Geometry: final body of the model. Coordinates: model frame, mm. Face numbers are marked on the shaded views. A direction names the side the tool comes from. Coordinates: 2 decimals unless noted, no trailing zeros. Order: outer loops, then holes, each group sorted by start corner. A loop starts at its lowest first (then second) coordinate and runs counter-clockwise, first axis right, second up. Notation, with made-up numbers: M 17.25,-25.5 L 27.25,-25.5 A26 ccw 27.25,-3.5 Z; hole C 48,40.5 d7. An arc over 180 degrees is marked long. Write item = value, one per line.
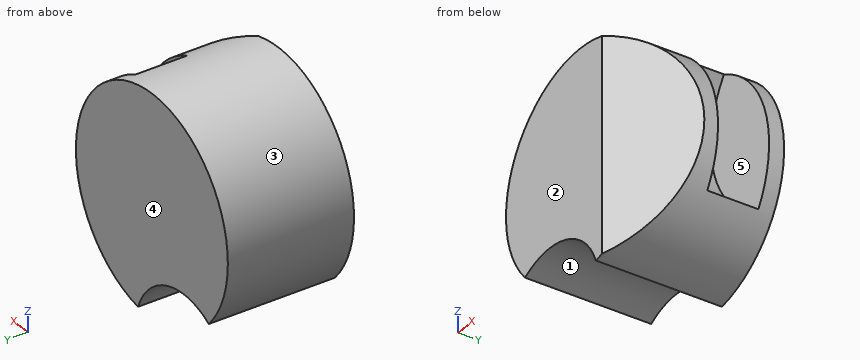
from build123d import *

# Parameters (mm, degrees)
BOSS_EXTRUDE1_DEPTH = 84
CUT_EXTRUDE2_DEPTH  = 34
CUT_EXTRUDE3_DEPTH  = 144.7823905
CUT_EXTRUDE4_DEPTH  = 43


with BuildPart() as part:
    # Sketch1 → Boss-Extrude1 (new body)
    with BuildSketch(Plane(origin=(0, 0, 0), x_dir=(1, 0, 0), z_dir=(0, 1, 0))):
        with BuildLine():
            ThreePointArc((-54.355236912, 47.976642444), (23.634324541, -68.539541168), (13.231432449, 71.2823905))
            ThreePointArc((13.231432449, 71.2823905), (-15.004428567, 43.512842845), (-54.355236912, 47.976642444))
        make_face()
    extrude(amount=BOSS_EXTRUDE1_DEPTH)

    # Sketch3 → Cut-Extrude2 (cut)
    with BuildSketch(Plane(origin=(0, 74, 0), x_dir=(1, 0, 0), z_dir=(0, 1, 0))):
        with BuildLine():
            ThreePointArc((62.290772837, 37.095951523), (20.191041077, -6.413624813), (29.465733324, -66.242135833))
            ThreePointArc((29.465733324, -66.242135833), (69.097787087, -21.948708839), (62.290772837, 37.095951523))
        make_face()
    extrude(amount=-CUT_EXTRUDE2_DEPTH, mode=Mode.SUBTRACT)

    # Sketch9 → Cut-Extrude3 (cut, through all)
    with BuildSketch(Plane.XY.offset(72.5)):
        Polygon((72.5, 30.908380348), (18.965114857, 0), (72.5, 0), align=None)
    extrude(amount=-CUT_EXTRUDE3_DEPTH, mode=Mode.SUBTRACT)

    # Sketch10 → Cut-Extrude4 (cut)
    with BuildSketch(Plane(origin=(0, 63, 0), x_dir=(1, 0, 0), z_dir=(0, 1, 0))):
        Polygon((-3.366442431, -32.270509831), (7.531695489, 1.270509831), (-21, 22), (-49.531695489, 1.270509831), (-38.633557569, -32.270509831), align=None)
    extrude(amount=-CUT_EXTRUDE4_DEPTH, mode=Mode.SUBTRACT)


solid = part.part
1) Mould query, pull axis X, two halves, no side actions, for the marked faces 1, 2 and 3. Classes: pulls with the +X half, pulls with the -X half, needs draft (parallel to the pull), parting line crosses it, or undercut.
Numbers:
face_1 = undercut
face_2 = needs draft
face_3 = parting line crosses it
2) Pin query (flat end, axial travel): pin 1 (2 mm diameter, centred on y = 66.5, z = -50, fed in from -X); pin 2 (17.5 mm diameter, centred on x = -23.5, y = 42, fed in from -Z); pin 3 (3 mm diameter, centred on x = 43.5, y = 47.5, fed in from -Z). Return the tip coordinate at first contact, or that it passes through.
Numbers:
pin_1 = -4.08
pin_2 = -43.6
pin_3 = -59.1
3) Section D-D, the plane x = 51. Return loops of the section in (y, z).
Numbers:
outline = M 18.5,-51.53 L 84,-51.53 L 84,51.53 L 74,51.53 L 74,-31.89 L 40,-31.89 L 40,51.53 L 18.5,51.53 Z
4) Set-up query: the marked faces 4 and 5. Return all of +Z, -Z, +X, -X, +Y, -Y with unobstructed straight access to the full face (end or side cutting, diameter ignored); none if empty.
Numbers:
face_4 = +Z, -Z, +X, -X, +Y
face_5 = +X
5) Section A-A, the plane x = 0. Return loops of the section in (y, z), and give its area (3 significant figures).
Numbers:
outline = M 0,-52.13 L 84,-52.13 L 84,72.5 L 0,72.5 Z; hole M 20,-6.74 L 63,-6.74 L 63,21.91 L 20,21.91 Z
area = 9,240 mm²
6) Section C-C, the plane z = 43. Return loops of the section in (x, y).
Numbers:
outline = M -58.37,0 L 18.97,0 L 58.37,22.75 L 58.37,40 L 18.91,40 L 18.91,74 L 58.37,74 L 58.37,84 L -58.37,84 Z
7) Line query: L1, parallel to Y at x = -29.5, z = -3; L2, parallel to Z at x = -9, y = 54; L3, parallel to X at y = 54.5, z = -17. Output: solid intervals per line, ascending.
Numbers:
L1 = 0 to 20, 63 to 84
L2 = -46.07 to -13.28, 32.27 to 71.94
L3 = -70.48 to -27.88, -14.12 to 33.15
8) Section B-B, the plane y = 44.5. Return loops of the section in (x, z).
Numbers:
outline = M -54.36,-47.98 A46 cw 13.23,-71.28 A72.5 ccw 62.29,-37.1 A68 cw 29.47,66.24 A72.5 ccw Z; hole M -49.53,-1.27 L -21,-22 L 7.53,-1.27 L -3.37,32.27 L -38.63,32.27 Z
